CAD build for the part. Positions are in the model's coordinates, mm. Face numbers are marked on the shaded views. A direction names the side the tool comes from. Give positions to 0.01 mm unless a question says otherwise; leave off trailing zeros. Write each loop counter-clockwise with the first axis right and the second up, starting at its lowest first coordinate (ties: lowest second). Pieces come first, ordered by that corner, then holes. Notation, with made-up numbers: (4, -30.75) - (12, -30.75) arc R11 cw to (12, -14.75) - close; hole circle Ø4 at (42.25, -0.5). An arc over 180 degrees is marked (long way). Write item = value, one per line. Start each with the question number.
```python
from build123d import *

# Parameters (mm, degrees)
F0_R     = 1.375
F1_DEPTH = 3
F2_R     = 1.375
F3_DEPTH = 1.5
F6_DEPTH = 26.3


with BuildPart() as f1:
    # F0 (on Front) → F1 (new body)
    with BuildSketch(Plane.XZ):
        with BuildLine():
            Line((9.087011, 12.915978), (-7.987775, 12.915978))
            ThreePointArc((-7.987775, 12.915978), (-11.523309, 11.451512), (-12.987775, 7.915978))
            Line((-12.987775, 7.915978), (-12.987775, -8.116753))
            Line((-12.987775, -8.116753), (-12.451817, -8.116753))
            Line((-12.451817, -8.116753), (13.087011, -8.116753))
            Line((13.087011, -8.116753), (13.087011, 8.915978))
            ThreePointArc((13.087011, 8.915978), (11.915438, 11.744405), (9.087011, 12.915978))
        make_face()
        with Locations((5.711206, -3.011084)):
            Circle(F0_R, mode=Mode.SUBTRACT)
        with BuildLine():
            Line((-9.236069, 8.065383), (-9.236069, 8.392912))
            Line((-9.236069, 8.392912), (-9.214787, 8.392912))
            ThreePointArc((-9.214787, 8.392912), (-6.705156, 10.596296), (-4.195525, 8.392912))
            Line((-4.195525, 8.392912), (-4.174243, 8.392912))
            Line((-4.174243, 8.392912), (-4.174243, 8.065383))
            Line((-4.174243, 8.065383), (-4.174243, 6.51706))
            Line((-4.174243, 6.51706), (-4.205156, 6.51706))
            ThreePointArc((-4.205156, 6.51706), (-6.705156, 4.01706), (-9.205156, 6.51706))
            Line((-9.205156, 6.51706), (-9.236069, 6.51706))
            Line((-9.236069, 6.51706), (-9.236069, 8.065383))
        make_face(mode=Mode.SUBTRACT)
        with Locations((5.711206, 6.427733)):
            Circle(F0_R, mode=Mode.SUBTRACT)
    extrude(amount=F1_DEPTH)

    # F2 (on face) → F3 (cut)
    with BuildSketch(Plane.XZ.offset(3)):
        with BuildLine():
            Line((8.118485, 10.503516), (3.118485, 10.503516))
            ThreePointArc((3.118485, 10.503516), (2.411378, 10.210622), (2.118485, 9.503516))
            Line((2.118485, 9.503516), (2.118485, -5.496484))
            ThreePointArc((2.118485, -5.496484), (2.411378, -6.203591), (3.118485, -6.496484))
            Line((3.118485, -6.496484), (8.118485, -6.496484))
            ThreePointArc((8.118485, -6.496484), (8.825592, -6.203591), (9.118485, -5.496484))
            Line((9.118485, -5.496484), (9.118485, 9.503516))
            ThreePointArc((9.118485, 9.503516), (8.825592, 10.210622), (8.118485, 10.503516))
        make_face()
        with Locations((5.711206, -3.011084)):
            Circle(F2_R, mode=Mode.SUBTRACT)
        with Locations((5.711206, 6.427733)):
            Circle(F2_R, mode=Mode.SUBTRACT)
    extrude(amount=-F3_DEPTH, mode=Mode.SUBTRACT)

    # F5 (on face) → F6 (join)
    with BuildSketch(Plane(origin=(-12.987775, 0, 0), x_dir=(0, -1, 0), z_dir=(-1, 0, 0))):
        with BuildLine():
            Line((0.094025, -8.107936), (0.023512, -9.205496))
            Line((0.023512, -9.205496), (2.672946, -11.868593))
            ThreePointArc((2.672946, -11.868593), (6.246579, -12.179247), (7.151377, -8.708124))
            ThreePointArc((7.151377, -8.708124), (6.782416, -8.293676), (6.249313, -8.139726))
            Line((6.249313, -8.139726), (5.643703, -8.139726))
            ThreePointArc((5.643703, -8.139726), (4.936596, -8.432619), (4.643703, -9.139726))
            Line((4.643703, -9.139726), (4.643703, -9.907948))
            Line((4.643703, -9.907948), (2.852926, -8.107936))
            Line((2.852926, -8.107936), (0.094025, -8.107936))
        make_face()
    extrude(amount=-F6_DEPTH)


solid = f1.part
```
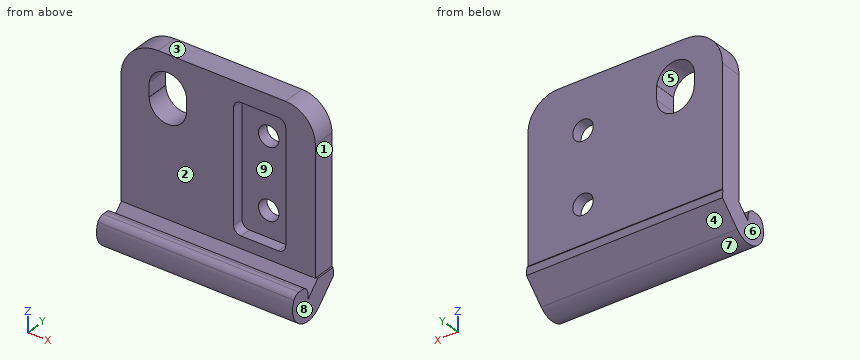
1. Mould opens along X. For the marked faces 6, 7, 8 and 9 say: +X half, -X half, draft (parallel to the pull), parting line (faces both ways), or undercut.
2. Cut at D-D (y = -3.75). Give the cut face in (x, z).
3. Cut at A-A (x = -8.75). Give the cut face in (y, z), then the cut area to 3 significant figures.
4. Cut at B-B (z = -1). Give the cut face in (x, y).
5. Wall check: line 1 along X through (y, z) = (-0.75, 2.5); line 2 along Y through (x, z) = (0, -6); line 3 along Y through (x, z) = (5.5, 1.5). Give the ranges that are in metal, low to high.
6. Tool access for the marked faces 1, 2, 3, 4 and 5: list every direction of +Z, -Z, +X, -X, +Y, -Y with a clear straight run to the whole face (end or side of a thin tool).
7. Cut at C-C (x = 4). Give the cut face in (y, z).
8. Pin check, flat tips, straight feed: pin 1 Ø8 at (x, z) = (-1.5, -2.5) entering from -Y; pin 2 Ø5 at (x, z) = (5, -6.5) entering from -Y; pin 3 Ø0.8 at (y, z) = (-2.5, 2.5) entering from +X; pin 4 Ø2 at (x, z) = (5.71, -3.01) entering from +Y. Stop position of each tip, or through.
Output:
q1.face_6 = -X half
q1.face_7 = draft
q1.face_8 = +X half
q1.face_9 = undercut
q2.outline = (-12.99, -12.54) - (13.31, -12.54) - (13.31, -9.01) - (-12.99, -9.01) - close
q3.outline = (-7.15, -8.71) arc R2.78 ccw to (-2.67, -11.87) - (-0.02, -9.21) - (-0.09, -8.12) - (0, -8.12) - (0, 5.08) - (-3, 5.08) - (-3, -8.12) - (-2.86, -8.12) - (-4.64, -9.91) - (-4.64, -9.14) arc R1 ccw to (-5.64, -8.14) - (-6.25, -8.14) arc R1 ccw to start; (-3, 9.56) - (0, 9.56) - (0, 12.86) - (-3, 12.86) - close
q3.area = 73.1 mm2
q4.outline = (-12.99, -3) - (2.12, -3) - (2.12, -1.5) - (9.12, -1.5) - (9.12, -3) - (13.09, -3) - (13.09, 0) - (-12.99, 0) - close
q5.line_1 = -12.99 to 13.09
q5.line_2 = -3 to 0
q5.line_3 = -1.5 to 0
q6.face_1 = +Z, +X, +Y, -Y
q6.face_2 = +Z, +X, -X, -Y
q6.face_3 = +Z, +X, -X, +Y, -Y
q6.face_4 = -Z, +X, -X, +Y
q6.face_5 = +Y, -Y
q7.outline = (-7.15, -8.71) arc R2.78 ccw to (-2.67, -11.87) - (-0.02, -9.21) - (-0.09, -8.12) - (0, -8.12) - (0, 12.92) - (-3, 12.92) - (-3, 10.5) - (-1.5, 10.5) - (-1.5, -6.5) - (-3, -6.5) - (-3, -8.12) - (-2.86, -8.12) - (-4.64, -9.91) - (-4.64, -9.14) arc R1 ccw to (-5.64, -8.14) - (-6.25, -8.14) arc R1 ccw to start
q8.pin_1 = -3
q8.pin_2 = -7.27
q8.pin_3 = 13.09
q8.pin_4 = through
